Source: CAD feature listing. Evaluate the final solid. Frame: model axes, mm. Round coordinates to 2 decimals unless told otherwise and drop trailing zeros. Loops run counter-clockwise (first coordinate to the right, second up) from the corner with the lowest first, then second, coordinate; pieces in that order, holes last. Notation, with made-up numbers: M -31,19 L 7,19 A31 cw 7,48 Z; hole C 70,37 d11. An arc over 180 degrees is marked long. Answer as a JSON object with one key per item and string values.
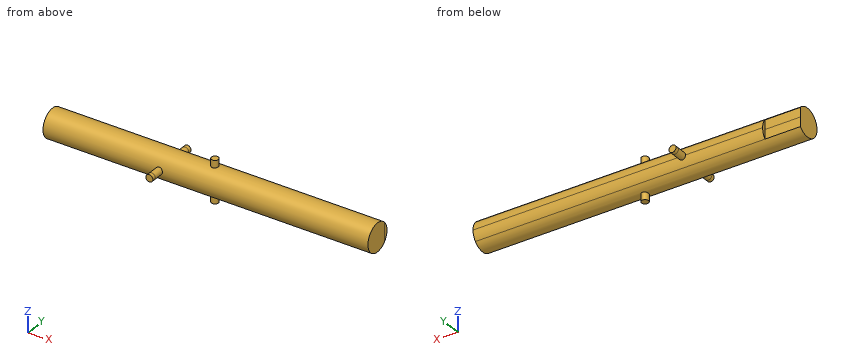
Autodesk Fusion 360 part; units mm, degrees
sketch "Esboço1" plane through (0, 0, 0) normal (1, 0, 0) x (0, 1, 0)
  circle A0 centre (0, 0) radius 4
  line L0 (0, 0) -> (3, 0) construction
  line L1 (3, 0) -> (3, -2.6458)
  line L2 (3, 0) -> (3, 2.6458)
  dimension "d1" = 8
  dimension "d2" = 3
extrude "Extrusão1" add sketch "Esboço1" along normal blind 92
extrude "Extrusão2" cut sketch "Esboço1" along normal blind 10 contours A0 L1 L2 picked at (3.6528, 0.1921)
sketch "Esboço2" plane through (0, 0, 0) normal (0, 1, 0) x (1, 0, 0)
sketch "Esboço3" plane through (0, 0, 0) normal (0, 0, 1) x (1, 0, 0)
  line L0 (0, 0) -> (46, 0) construction
  circle A0 centre (46, 0) radius 1
  dimension "d7" = 46
  dimension "d24" = 2
sketch "Esboço4" plane through (0, 0, 0) normal (0, 1, 0) x (1, 0, 0)
  line L0 (92, 0) -> (32.816, 0) construction
  circle A0 centre (32.816, 0) radius 1
  dimension "d13" = 59.184
  dimension "d23" = 2
extrude "Extrusão7" add sketch "Esboço3" along normal blind 6 and the other way blind 6
extrude "Extrusão8" add sketch "Esboço4" along normal blind 7 and the other way blind 7
extrude "Extrusão9" add 1 faces at (32.4233, -7, 0.2267) along direction (0, -1, 0) blind 1
extrude "Extrusão10" add 1 faces at (32.4233, 7, 0.2267) along direction (0, 1, 0) blind 1
sketch "Esboço5" plane through (0, -8, 0) normal (0, -1, 0) x (1, 0, 0)
  circle A0 centre (32.816, 0) radius 1
equation "d13 = 58.434 mm + 0.75 mm"
Item 1: Section B-B on y = 0. Return the cut outline in (x, z), then the cut area to 3 significant figures.
Answer sheet:
{"outline": "M 0,-4 L 45,-4 L 45,-6 L 47,-6 L 47,-4 L 92,-4 L 92,4 L 47,4 L 47,6 L 45,6 L 45,4 L 0,4 Z", "area": "744 mm²"}
Item 2: Section D-D on x = 85. Return the cut outline in (y, z).
Answer sheet:
{"outline": "C 0,0 d8"}
Item 3: Section C-C on z = -5. Return the cut outline in (x, y), then the cut area to 3 significant figures.
Answer sheet:
{"outline": "C 46,0 d2", "area": "3.14 mm²"}
Item 4: Contact query for flat-ended pins moving along their axis: pin 1 Ø2 at (x, z) = (6, 1) entering from +Y; pin 2 Ø3 at (x, z) = (72.5, -1.5) entering from -Y; pin 3 Ø2 at (x, y) = (46.5, -3.5) entering from -Z. Output: stop coordinate, or through.
Answer sheet:
{"pin 1": "stops at y = 3", "pin 2": "stops at y = -4", "pin 3": "stops at z = -3.12"}
Item 5: Line query: probe 1 along Y at (x, z) = (31.5, 0); probe 2 along Z at (x, y) = (37, 3); probe 3 along X at (y, z) = (-0.75, 4.25). Output: solid intervals per line, ascending. Write a range as from..to.
Answer sheet:
{"probe 1": "y = -4..4", "probe 2": "z = -2.65..2.65", "probe 3": "x = 45.34..46.66"}
Item 6: Section A-A on x = 46. Return the cut outline in (y, z).
Answer sheet:
{"outline": "M -1,-6 L 1,-6 L 1,-3.87 A4 ccw 1,3.87 L 1,6 L -1,6 L -1,3.87 A4 ccw -1,-3.87 Z"}
